from build123d import *

# Parameters (mm, degrees)
BOSS_EXTRUDE1_DEPTH = 19.5
BOSS_EXTRUDE5_DEPTH = 1.5
BOSS_EXTRUDE6_DEPTH = 1.5
SKETCH8_R           = 6.75
CUT_EXTRUDE2_DEPTH  = 35.70752685
BOSS_EXTRUDE7_DEPTH = 2.5
SKETCH10_R          = 1.75
BOSS_EXTRUDE8_DEPTH = 5
CHAMFER1_SIZE       = 1.5
CHAMFER2_SIZE       = 1
SKETCH11_R          = 2.875
SKETCH11_R_2        = 1.75
CUT_EXTRUDE4_DEPTH  = 2.5
REVOLVE1_ANGLE      = 180
CHAMFER3_SIZE       = 1


with BuildPart() as part:
    # Sketch1 → Boss-Extrude1 (new body)
    with BuildSketch(Plane.XY):
        Polygon((-11.779, -12.684829289), (-10.279, -12.684829289), (-10.279, -0.473504424), (-11.944063509, 0.487820441), (-11.944063509, 1.64252098), (-9.912974596, 2.815170711), (-9.427494989, 2.815170711), (-9.427494989, 4.973204454), (-6.75, 9.910826582), (0, 9.910826582), (0, 12.684829289), (-7.456216647, 12.684829289), (-13.444063509, 1.64252098), (-13.444063509, 0.487820441), align=None)
    extrude(amount=BOSS_EXTRUDE1_DEPTH)

    # Sketch6 → Boss-Extrude5 (add)
    with BuildSketch(Plane.XY.offset(19.5)):
        Polygon((0, 12.684829289), (-7.456216647, 12.684829289), (-13.444063509, 1.64252098), (-13.444063509, 0.487820441), (-11.779, -12.684829289), (0, -12.684829289), align=None)
    extrude(amount=-BOSS_EXTRUDE5_DEPTH)

    # Sketch7 → Boss-Extrude6 (add)
    with BuildSketch(Plane(origin=(0, 0, 0), x_dir=(-1, 0, 0), z_dir=(0, 0, -1))):
        Polygon((0, 12.684829289), (0, -12.684829289), (11.779, -12.684829289), (13.444063509, 0.487820441), (13.444063509, 1.64252098), (7.456216647, 12.684829289), align=None)
    extrude(amount=-BOSS_EXTRUDE6_DEPTH)

    # Sketch8 → Cut-Extrude2 (cut, through all)
    with BuildSketch(Plane(origin=(0, 12.684829289, 0), x_dir=(1, 0, 0), z_dir=(0, 1, 0))):
        with Locations((0, -9.75)):
            Circle(SKETCH8_R)
    extrude(amount=-CUT_EXTRUDE2_DEPTH, mode=Mode.SUBTRACT)

    # Sketch9 → Boss-Extrude7 (add, symmetric)
    with BuildSketch(Plane(origin=(0, 12.684829289, 0), x_dir=(1, 0, 0), z_dir=(0, 1, 0))):
        with BuildLine():
            Line((0, -1.5), (0, -3))
            ThreePointArc((0, -3), (-6.75, -9.75), (0, -16.5))
            Line((0, -16.5), (0, -18))
            ThreePointArc((0, -18), (-8.25, -9.75), (0, -1.5))
        make_face()
    extrude(amount=BOSS_EXTRUDE7_DEPTH, both=True)

    # Sketch10 → Boss-Extrude8 (add)
    with BuildSketch(Plane(origin=(0, 0, 0), x_dir=(0, 0, -1), z_dir=(1, 0, 0))):
        Polygon((-19.5, 12.684829289), (-27.043783602, 4.79693847), (-27.043783602, -4.79693847), (-19.5, -12.684829289), align=None)
        Polygon((-20.396891801, -1.659882024), (-20.396891801, 1.659882024), (-23.271891801, 3.319764048), (-26.146891801, 1.659882024), (-26.146891801, -1.659882024), (-23.271891801, -3.319764048), align=None, mode=Mode.SUBTRACT)
        Polygon((-23.271891801, -3.319764048), (-20.396891801, -1.659882024), (-20.396891801, 1.659882024), (-23.271891801, 3.319764048), (-26.146891801, 1.659882024), (-26.146891801, -1.659882024), align=None)
        with Locations(Location((-23.271891801, 0, 0), (0, 0, 90))):
            Circle(SKETCH10_R, mode=Mode.SUBTRACT)
        Polygon((7.543783602, 4.79693847), (0, 12.684829289), (0, -12.684829289), (7.543783602, -4.79693847), align=None)
        Polygon((6.646891801, 1.659882024), (3.771891801, 3.319764048), (0.896891801, 1.659882024), (0.896891801, -1.659882024), (3.771891801, -3.319764048), (6.646891801, -1.659882024), align=None, mode=Mode.SUBTRACT)
        Polygon((6.646891801, 1.659882024), (6.646891801, -1.659882024), (3.771891801, -3.319764048), (0.896891801, -1.659882024), (0.896891801, 1.659882024), (3.771891801, 3.319764048), align=None)
        with Locations(Location((3.771891801, 0, 0), (0, 0, 90))):
            Circle(SKETCH10_R, mode=Mode.SUBTRACT)
    extrude(amount=-BOSS_EXTRUDE8_DEPTH)

    # Chamfer1
    chamfer1_edges = [part.edges().sort_by_distance(p)[0] for p in [
        (-12.611531755, -6.098504424, 19.5),
        (-13.444063509, 1.065170711, 19.5),
        (-10.450140078, 7.163675135, 19.5),
        (-12.611531755, -6.098504424, 0),
        (-13.444063509, 1.065170711, 0),
        (-10.450140078, 7.163675135, 0),
    ]]
    chamfer(chamfer1_edges, length=CHAMFER1_SIZE)

    # Chamfer2
    chamfer2_edges = [part.edges().sort_by_distance(p)[0] for p in [
        (-8.25, 15.184829289, 9.75),
    ]]
    chamfer(chamfer2_edges, length=CHAMFER2_SIZE)

    # Sketch11 → Cut-Extrude4 (cut)
    with BuildSketch(Plane.ZY.offset(5)):
        with Locations(Location((-3.771891801, 0, 0), (0, 0, 270))):
            Circle(SKETCH11_R)
        with Locations(Location((-3.771891801, 0, 0), (0, 0, 90))):
            Circle(SKETCH11_R_2, mode=Mode.SUBTRACT)
        with Locations(Location((23.271891801, 0, 0), (0, 0, 270))):
            Circle(SKETCH11_R)
        with Locations(Location((23.271891801, 0, 0), (0, 0, 90))):
            Circle(SKETCH11_R_2, mode=Mode.SUBTRACT)
    extrude(amount=-CUT_EXTRUDE4_DEPTH, mode=Mode.SUBTRACT)

    # Sketch12 → Revolve1 (revolve)
    with BuildSketch(Plane(origin=(0, 0, 0), x_dir=(0, 0, -1), z_dir=(1, 0, 0))):
        Polygon((-16.5, 15.184829289), (-16.5, 14.184829289), (-15.75, 14.684829289), align=None)
    revolve(axis=Axis((0, 15.184829289, 9.75), (0, -1, 0)), revolution_arc=REVOLVE1_ANGLE)

    # Chamfer3
    chamfer3_edges = [part.edges().sort_by_distance(p)[0] for p in [
        (-4.412056396, 12.684829289, 2.77889834),
        (-4.412056396, 12.684829289, 16.72110166),
    ]]
    chamfer(chamfer3_edges, length=CHAMFER3_SIZE)


solid = part.part
Verification items for the finished model (mm, model axes). A direction names the side the tool comes from. Give positions to 0.01 mm unless a question says otherwise; leave off trailing zeros. Write each loop counter-clockwise with the first axis right and the second up, starting at its lowest first coordinate (ties: lowest second). Pieces come first, ordered by that corner, then holes. Notation, with made-up numbers: (89, -18.75) -> (97, -18.75) arc R13 ccw to (97, -0.75) -> close; hole circle Ø4 at (67.5, -2.5). An arc over 180 degrees is marked (long way). Use CSV: the item, a comma, the result in double quotes.
(1) Release check for a two-part mould opening along Z. For faces 4 (the flat face through (-12.623, -6.006, 9.634)), 5 (the flat face through (-8.107, 7.407, 9.634)), 6 (the flat face through (-8, -3, 19.5)), 7 (the cylindrical face through (-6.75, 12.08, 9.6)) record: +Z half, -Z half, draft (parallel to the pull), parting line (faces both ways), or undercut.
Derived:
face 4,"draft"
face 5,"undercut"
face 6,"+Z half"
face 7,"undercut"
(2) Go/stop test with flat-tipped pins: pin 1 (10 mm diameter, centred on y = 12, z = 13.5, fed in from -X); pin 2 (4.5 mm diameter, centred on y = -0.5, z = 24, fed in from -X); pin 3 (1 mm diameter, centred on x = -6.5, z = 3, fed in from -Y). Record where each tip stops, or that it passes through.
Derived:
pin 1,"stops at x = -10.54"
pin 2,"stops at x = -5"
pin 3,"stops at y = 9.45"
(3) Material ranges on L1, parallel to Z at x = -3.6, y = 0; L2, parallel to Z at x = -0.9, y = 0; L3, parallel to Z at x = -3.5, y = -3.5, recorded low to high.
Derived:
L1,"z = -7.54 to -6.65, -0.9 to 1.5, 18 to 20.4, 26.15 to 27.04"
L2,"z = -7.54 to -5.52, -2.02 to 1.5, 18 to 21.52, 25.02 to 27.04"
L3,"z = -7.54 to 1.5, 18 to 27.04"
(4) Sectioned sample at A-A (y = 0). Give the number of separate pieces and of enclosed holes in the cut face, plus the area to 3 significant figures.
Derived:
separate pieces,"3"
enclosed holes,"0"
area,"105 mm^2"
(5) Set-up check for faces 1 (the flat face through (-5, 0.2, -0.4)), 2 (the flat face through (-2.5, -2, 23)), 3 (the flat face through (-5, 12.685, 1)): record each of +Z, -Z, +X, -X, +Y, -Y from which the full face is reachable in a straight line by a thin tool's end or side.
Derived:
face 1,"-Z, -X, +Y, -Y"
face 2,"-X"
face 3,"-Z, -X, +Y"
(6) Sectioned sample at C-C (y = -8.75). Record the cut outline in (x, z).
Derived:
outline,"(-12.28, 1.5) -> (-10.76, 0) -> (-5, 0) -> (-5, -3.76) -> (0, -3.76) -> (0, 1.5) -> (-10.28, 1.5) -> (-10.28, 18) -> (0, 18) -> (0, 23.26) -> (-5, 23.26) -> (-5, 19.5) -> (-10.76, 19.5) -> (-12.28, 18) -> close"
